Design review of the part built by this model. Coordinates are the model's own, in mm. A direction names the side the tool comes from. Round coordinates to 2 decimals unless told otherwise and drop trailing zeros. Write each loop counter-clockwise with the first axis right and the second up, starting at its lowest first coordinate (ties: lowest second). Pieces come first, ordered by that corner, then holes. Notation, with made-up numbers: (75, -13.5) -> (79, -13.5) arc R11 cw to (79, -3.5) -> close; hole circle Ø9 at (50.25, 8.5). An arc over 180 degrees is marked (long way). Write item = value, one per line. Start each with the question number.
Item 1: Add section A-A, the plane x = 31.5. State the section outline as (y, z) points, then the cut area to 3 significant figures.
Item 2: Add section B-B, the plane y = 3.5. State how many separate pieces and enclosed holes the cut face has, then the cut area to 3 significant figures.
Item 3: For pin 1 Ø2 at (x, y) = (25, 2.5) entering from -Z; pin 2 Ø6.5 at (x, z) = (0, 0) entering from +Y; pin 3 Ø2 at (x, z) = (30.75, 0) entering from -Y; pin 4 Ø1 at (x, y) = (16.5, 4.5) entering from +Z, all flat-tipped, find the tip position at first contact; note any pin that passes through.
Item 4: Add section C-C, the plane x = 21. State the section outline as (y, z) points.
Item 5: Mouldability with a two-part tool opening along Z and no side actions: class faces 4 (the cylindrical face through (-5.98, 3.451, 12.023)), 5 (the cylindrical face through (29.2, 3.45, 0.81)), 6 (the cylindrical face through (-5.952, 3.451, -11.996)) as released by +Z, released by -Z, zero draft, split by the parting line, or undercut.
Item 6: To check wall thickness, follow L1, parallel to X at y = 4, z = 0; L2, parallel to X at y = 1.6, z = 0; L3, parallel to Z at x = 9, y = 3.5. State the ranges of each line that lie inside material, in increasing order.
Item 7: Machinability: for faces 1 (the cylindrical face through (-4.273, 3.451, -12.73)), 2 (the cylindrical face through (-8.888, 3.451, 10.066)), 3 (the cylindrical face through (-11.988, 3.451, 1.571)), which of the approach directions +Z, -Z, +X, -X, +Y, -Y give a long, thin tool a straight path to every point of the face, cutting with its end or side? Answer none if there is none.
Item 8: Add section D-D, the plane z = -6. State the section outline as (x, y) points, then the cut area to 3 significant figures.
from build123d import *

# Parameters (mm, degrees)
SKETCH1_R           = 3.5
SKETCH1_R_2         = 1.75
BOSS_EXTRUDE1_DEPTH = 7
SKETCH2_R           = 3.5
SKETCH2_R_2         = 1.75
BOSS_EXTRUDE2_DEPTH = 2


with BuildPart() as part:
    # Sketch1 → Boss-Extrude1 (new body)
    with BuildSketch(Plane(origin=(0, 0, 0), x_dir=(1, 0, 0), z_dir=(0, 1, 0))):
        with BuildLine():
            ThreePointArc((1.04, 12.04518576), (0.838273314, 13.383704325), (0.31, 14.63))
            Line((0.31, 14.63), (-0.31, 14.63))
            ThreePointArc((-0.31, 14.63), (-0.838273314, 13.383704325), (-1.04, 12.04518576))
            ThreePointArc((-1.04, 12.04518576), (-1.578061664, 11.986568374), (-2.112960617, 11.903927815))
            ThreePointArc((-2.112960617, 11.903927815), (-2.65424773, 13.144626757), (-3.487085624, 14.211728743))
            Line((-3.487085624, 14.211728743), (-4.085959636, 14.051260935))
            ThreePointArc((-4.085959636, 14.051260935), (-4.273667417, 12.71070456), (-4.122086336, 11.365584201))
            ThreePointArc((-4.122086336, 11.365584201), (-4.626642697, 11.169703548), (-5.12192646, 10.951436862))
            ThreePointArc((-5.12192646, 10.951436862), (-5.965886177, 12.009764599), (-7.046532125, 12.824951657))
            Line((-7.046532125, 12.824951657), (-7.583467875, 12.514951657))
            ThreePointArc((-7.583467875, 12.514951657), (-7.417818147, 11.171491285), (-6.9232593, 9.911436862))
            ThreePointArc((-6.9232593, 9.911436862), (-7.359925677, 9.591641884), (-7.781841479, 9.252623584))
            ThreePointArc((-7.781841479, 9.252623584), (-8.870959341, 10.05645683), (-10.125769107, 10.564175311))
            Line((-10.125769107, 10.564175311), (-10.564175311, 10.125769107))
            ThreePointArc((-10.564175311, 10.125769107), (-10.05645683, 8.870959341), (-9.252623584, 7.781841479))
            ThreePointArc((-9.252623584, 7.781841479), (-9.591641884, 7.359925677), (-9.911436862, 6.9232593))
            ThreePointArc((-9.911436862, 6.9232593), (-11.171491285, 7.417818147), (-12.514951657, 7.583467875))
            Line((-12.514951657, 7.583467875), (-12.824951657, 7.046532125))
            ThreePointArc((-12.824951657, 7.046532125), (-12.009764599, 5.965886177), (-10.951436862, 5.12192646))
            ThreePointArc((-10.951436862, 5.12192646), (-11.169703548, 4.626642697), (-11.365584201, 4.122086336))
            ThreePointArc((-11.365584201, 4.122086336), (-12.71070456, 4.273667417), (-14.051260935, 4.085959636))
            Line((-14.051260935, 4.085959636), (-14.211728743, 3.487085624))
            ThreePointArc((-14.211728743, 3.487085624), (-13.144626757, 2.65424773), (-11.903927815, 2.112960617))
            ThreePointArc((-11.903927815, 2.112960617), (-11.986568374, 1.578061664), (-12.04518576, 1.04))
            ThreePointArc((-12.04518576, 1.04), (-13.383704325, 0.838273314), (-14.63, 0.31))
            Line((-14.63, 0.31), (-14.63, -0.31))
            ThreePointArc((-14.63, -0.31), (-13.383704325, -0.838273314), (-12.04518576, -1.04))
            ThreePointArc((-12.04518576, -1.04), (-11.986568374, -1.578061664), (-11.903927815, -2.112960617))
            ThreePointArc((-11.903927815, -2.112960617), (-13.144626757, -2.65424773), (-14.211728743, -3.487085624))
            Line((-14.211728743, -3.487085624), (-14.051260935, -4.085959636))
            ThreePointArc((-14.051260935, -4.085959636), (-12.71070456, -4.273667417), (-11.365584201, -4.122086336))
            ThreePointArc((-11.365584201, -4.122086336), (-11.169703548, -4.626642697), (-10.951436862, -5.12192646))
            ThreePointArc((-10.951436862, -5.12192646), (-12.009764599, -5.965886177), (-12.824951657, -7.046532125))
            Line((-12.824951657, -7.046532125), (-12.514951657, -7.583467875))
            ThreePointArc((-12.514951657, -7.583467875), (-11.171491285, -7.417818147), (-9.911436862, -6.9232593))
            ThreePointArc((-9.911436862, -6.9232593), (-9.591641884, -7.359925677), (-9.252623584, -7.781841479))
            ThreePointArc((-9.252623584, -7.781841479), (-10.05645683, -8.870959341), (-10.564175311, -10.125769107))
            Line((-10.564175311, -10.125769107), (-10.125769107, -10.564175311))
            ThreePointArc((-10.125769107, -10.564175311), (-8.870959341, -10.05645683), (-7.781841479, -9.252623584))
            ThreePointArc((-7.781841479, -9.252623584), (-7.359925677, -9.591641884), (-6.9232593, -9.911436862))
            ThreePointArc((-6.9232593, -9.911436862), (-7.417818147, -11.171491285), (-7.583467875, -12.514951657))
            Line((-7.583467875, -12.514951657), (-7.046532125, -12.824951657))
            ThreePointArc((-7.046532125, -12.824951657), (-5.965886177, -12.009764599), (-5.12192646, -10.951436862))
            ThreePointArc((-5.12192646, -10.951436862), (-4.626642697, -11.169703548), (-4.122086336, -11.365584201))
            ThreePointArc((-4.122086336, -11.365584201), (-4.273667417, -12.71070456), (-4.085959636, -14.051260935))
            Line((-4.085959636, -14.051260935), (-3.487085624, -14.211728743))
            ThreePointArc((-3.487085624, -14.211728743), (-2.65424773, -13.144626757), (-2.112960617, -11.903927815))
            ThreePointArc((-2.112960617, -11.903927815), (-1.578061664, -11.986568374), (-1.04, -12.04518576))
            ThreePointArc((-1.04, -12.04518576), (-0.838273314, -13.383704325), (-0.31, -14.63))
            Line((-0.31, -14.63), (0.31, -14.63))
            ThreePointArc((0.31, -14.63), (0.838273314, -13.383704325), (1.04, -12.04518576))
            ThreePointArc((1.04, -12.04518576), (1.578061664, -11.986568374), (2.112960617, -11.903927815))
            ThreePointArc((2.112960617, -11.903927815), (2.65424773, -13.144626757), (3.487085624, -14.211728743))
            Line((3.487085624, -14.211728743), (4.085959636, -14.051260935))
            ThreePointArc((4.085959636, -14.051260935), (4.273667417, -12.71070456), (4.122086336, -11.365584201))
            ThreePointArc((4.122086336, -11.365584201), (4.626642697, -11.169703548), (5.12192646, -10.951436862))
            ThreePointArc((5.12192646, -10.951436862), (5.965886177, -12.009764599), (7.046532125, -12.824951657))
            Line((7.046532125, -12.824951657), (7.583467875, -12.514951657))
            ThreePointArc((7.583467875, -12.514951657), (7.417818147, -11.171491285), (6.9232593, -9.911436862))
            ThreePointArc((6.9232593, -9.911436862), (7.359925677, -9.591641884), (7.781841479, -9.252623584))
            ThreePointArc((7.781841479, -9.252623584), (8.870959341, -10.05645683), (10.125769107, -10.564175311))
            Line((10.125769107, -10.564175311), (10.564175311, -10.125769107))
            ThreePointArc((10.564175311, -10.125769107), (10.05645683, -8.870959341), (9.252623584, -7.781841479))
            ThreePointArc((9.252623584, -7.781841479), (9.591641884, -7.359925677), (9.911436862, -6.9232593))
            ThreePointArc((9.911436862, -6.9232593), (11.171491285, -7.417818147), (12.514951657, -7.583467875))
            Line((12.514951657, -7.583467875), (12.824951657, -7.046532125))
            ThreePointArc((12.824951657, -7.046532125), (12.009764599, -5.965886177), (10.951436862, -5.12192646))
            ThreePointArc((10.951436862, -5.12192646), (11.194344337, -4.566700654), (11.409123542, -4))
            Line((11.409123542, -4), (30.75, -4))
            ThreePointArc((30.75, -4), (34.75, 0), (30.75, 4))
            Line((30.75, 4), (11.409123542, 4))
            ThreePointArc((11.409123542, 4), (11.194344337, 4.566700654), (10.951436862, 5.12192646))
            ThreePointArc((10.951436862, 5.12192646), (12.009764599, 5.965886177), (12.824951657, 7.046532125))
            Line((12.824951657, 7.046532125), (12.514951657, 7.583467875))
            ThreePointArc((12.514951657, 7.583467875), (11.171491285, 7.417818147), (9.911436862, 6.9232593))
            ThreePointArc((9.911436862, 6.9232593), (9.591641884, 7.359925677), (9.252623584, 7.781841479))
            ThreePointArc((9.252623584, 7.781841479), (10.05645683, 8.870959341), (10.564175311, 10.125769107))
            Line((10.564175311, 10.125769107), (10.125769107, 10.564175311))
            ThreePointArc((10.125769107, 10.564175311), (8.870959341, 10.05645683), (7.781841479, 9.252623584))
            ThreePointArc((7.781841479, 9.252623584), (7.359925677, 9.591641884), (6.9232593, 9.911436862))
            ThreePointArc((6.9232593, 9.911436862), (7.417818147, 11.171491285), (7.583467875, 12.514951657))
            Line((7.583467875, 12.514951657), (7.046532125, 12.824951657))
            ThreePointArc((7.046532125, 12.824951657), (5.965886177, 12.009764599), (5.12192646, 10.951436862))
            ThreePointArc((5.12192646, 10.951436862), (4.626642697, 11.169703548), (4.122086336, 11.365584201))
            ThreePointArc((4.122086336, 11.365584201), (4.273667417, 12.71070456), (4.085959636, 14.051260935))
            Line((4.085959636, 14.051260935), (3.487085624, 14.211728743))
            ThreePointArc((3.487085624, 14.211728743), (2.65424773, 13.144626757), (2.112960617, 11.903927815))
            ThreePointArc((2.112960617, 11.903927815), (1.578061664, 11.986568374), (1.04, 12.04518576))
        make_face()
        with Locations(Location((0, 0, 0), (0, 0, 270))):
            Circle(SKETCH1_R, mode=Mode.SUBTRACT)
        with Locations(Location((30.75, 0, 0), (0, 0, 270))):
            Circle(SKETCH1_R_2, mode=Mode.SUBTRACT)
    extrude(amount=BOSS_EXTRUDE1_DEPTH)

    # Sketch2 → Boss-Extrude2 (add)
    with BuildSketch(Plane.XZ):
        with Locations(Location((0, 0, 0), (0, 0, 270))):
            Circle(SKETCH2_R)
        with Locations(Location((0, 0, 0), (0, 0, 270))):
            Circle(SKETCH2_R_2, mode=Mode.SUBTRACT)
    extrude(amount=-BOSS_EXTRUDE2_DEPTH)


solid = part.part
Result set:
q1.outline = (0, -3.93) -> (7, -3.93) -> (7, -1.58) -> (0, -1.58) -> close; (0, 1.58) -> (7, 1.58) -> (7, 3.93) -> (0, 3.93) -> close
q1.area = 32.9 mm²
q2.separate_pieces = 1
q2.enclosed_holes = 2
q2.area = 672 mm²
q3.pin_1 = -4
q3.pin_2 = 2
q3.pin_3 = through
q3.pin_4 = 4
q4.outline = (0, -4) -> (7, -4) -> (7, 4) -> (0, 4) -> close
q5.face_4 = released by +Z
q5.face_5 = undercut
q5.face_6 = released by -Z
q6.L1 = -14.63 to -3.5, 3.5 to 29, 32.5 to 34.75
q6.L2 = -14.63 to -1.75, 1.75 to 29, 32.5 to 34.75
q6.L3 = -10.13 to 10.13
q7.face_1 = +Y, -Y
q7.face_2 = +Z, +Y, -Y
q7.face_3 = -X, +Y, -Y
q8.outline = (-12.04, 0) -> (12.04, 0) -> (12.04, 7) -> (-12.04, 7) -> close
q8.area = 169 mm²
